Autodesk Inventor part; units mm, degrees
ref_plane "YZ Plane" through (0, 0, 0) normal (1, 0, 0) x (0, 1, 0)
ref_plane "XZ Plane" through (0, 0, 0) normal (0, 1, 0) x (-1, 0, 0)
ref_plane "XY Plane" through (0, 0, 0) normal (0, 0, 1) x (1, 0, 0)
sketch "Sketch1" plane through (0, 0, 0) normal (0, 0, 1) x (1, 0, 0)
  line L0 (0, 0) -> (1219.2, 0)
  line L1 (1219.2, 0) -> (1219.2, 609.6)
  line L2 (1219.2, 609.6) -> (0, 609.6)
  line L3 (0, 609.6) -> (0, 0)
  dimension "d0" = 1219.2
  dimension "d1" = 609.6
extrude "Extrusion1" add sketch "Sketch1" along normal blind 15.875
sketch "Sketch2" plane through (0, 0, 15.875) normal (0, 0, 1) x (1, 0, 0)
  line L0 (342.9, 228.6) -> (419.1, 228.6)
  line L1 (419.1, 228.6) -> (419.1, 304.8)
  line L2 (419.1, 304.8) -> (342.9, 304.29)
  line L3 (342.9, 304.29) -> (342.9, 228.6)
  line L4 (876.3, 228.6) -> (876.3, 304.8)
  line L5 (876.3, 304.8) -> (800.1, 304.8)
  line L6 (800.1, 304.8) -> (800.1, 228.6)
  line L7 (800.1, 228.6) -> (876.3, 228.6)
  dimension "d13" = 76.2
  dimension "d15" = 76.2
  dimension "d16" = 76.2
  dimension "d17" = 76.2
extrude "Extrusion2" cut sketch "Sketch2" against normal blind 15.875
properties part number "model 1 window board"
Could you check a few things on this model? Use its own coordinates, in mm. Round coordinates to 2 decimals unless told otherwise and drop trailing zeros. Write each loop counter-clockwise with the first axis right and the second up, starting at its lowest first coordinate (ties: lowest second). Pieces come first, ordered by that corner, then holes. Notation, with made-up numbers: (-22, 75) - (13, 75) arc R8 cw to (13, 80) - close; hole circle Ø2 at (1, 25). An arc over 180 degrees is marked (long way). Put each result on its own line as item: value. Start each with the question number.
(1) I want a section at A-A, the plane z = 11. Please give me the cut outline in (x, y), plus the area to 3 significant figures.
(2) I need wall thicknesses on probe 1 along X at (y, z) = (248.5, 2.75); probe 2 along Y at (x, z) = (364, 4.5); probe 3 along Y at (x, z) = (847.5, 11). Which ranges of each line are inside material? Lowest first, please.
(3) Will this pin go through, and if not, where does the flat tip stop? pin 1 (5 mm diameter, centred on y = 502.5, z = 10.5, fed in from -X).
(4) I want a section at B-B, the plane x = 815. Please give me the cut outline in (y, z) (3 decimals), plus the area to 3 significant figures.
Here are the results:
1. outline: (0, 0) - (1219.2, 0) - (1219.2, 609.6) - (0, 609.6) - close; hole (342.9, 228.6) - (419.1, 228.6) - (419.1, 304.8) - (342.9, 304.29) - close; hole (800.1, 228.6) - (876.3, 228.6) - (876.3, 304.8) - (800.1, 304.8) - close
1. area: 732,000 mm^2
2. probe 1: x = 0 to 342.9, 419.1 to 800.1, 876.3 to 1219.2
2. probe 2: y = 0 to 228.6, 304.43 to 609.6
2. probe 3: y = 0 to 228.6, 304.8 to 609.6
3. pin 1: stops at x = 0
4. outline: (0, 0) - (228.6, 0) - (228.6, 15.875) - (0, 15.875) - close; (304.8, 0) - (609.6, 0) - (609.6, 15.875) - (304.8, 15.875) - close
4. area: 8,470 mm^2
